```python
from build123d import *

# Parameters (mm, degrees)
F0_R     = 4.925
F0_W     = 15.85
F0_H     = 3
F0_H_2   = 14
F1_DEPTH = 3
F2_DEPTH = 60
F3_DEPTH = 10


with BuildPart() as f1:
    # F0 (on Top) → F1 (new body)
    with BuildSketch(Plane.XY):
        with BuildLine():
            Line((-7.925, 5.925), (-7.925, 0))
            ThreePointArc((-7.925, 0), (0, -7.925), (7.925, 0))
            Line((7.925, 0), (7.925, 5.925))
            Line((7.925, 5.925), (-7.925, 5.925))
        make_face()
        Circle(F0_R, mode=Mode.SUBTRACT)
        with Locations((0, 7.425)):
            Rectangle(F0_W, F0_H)
        with Locations((0, 15.925)):
            Rectangle(F0_W, F0_H_2)
        with Locations((0, 24.425)):
            Rectangle(F0_W, F0_H)
    extrude(amount=F1_DEPTH)

    # F0 (on Top) → F2 (join)
    with BuildSketch(Plane.XY):
        with Locations((0, 7.425)):
            Rectangle(F0_W, F0_H)
        with Locations((0, 24.425)):
            Rectangle(F0_W, F0_H)
    extrude(amount=F2_DEPTH)

    # F0 (on Top) → F3 (join)
    with BuildSketch(Plane.XY):
        with BuildLine():
            Line((-7.925, 5.925), (-7.925, 0))
            ThreePointArc((-7.925, 0), (0, -7.925), (7.925, 0))
            Line((7.925, 0), (7.925, 5.925))
            Line((7.925, 5.925), (-7.925, 5.925))
        make_face()
        Circle(F0_R, mode=Mode.SUBTRACT)
    extrude(amount=F3_DEPTH)


solid = f1.part
```
Geometry: final body of the model. Coordinates: model frame, mm. A direction names the side the tool comes from. Give positions to 0.01 mm unless a question says otherwise; leave off trailing zeros. Loops run counter-clockwise (first coordinate to the right, second up) from the corner with the lowest first, then second, coordinate; pieces in that order, holes last. Notation, with made-up numbers: (15, 39) - (20, 39) arc R33 ccw to (20, 72) - close; hole circle Ø11 at (56, 15.5). An arc over 180 degrees is marked (long way). Answer as CSV lines item,"result". Start each with the question number.
(1) Section query B-B (x = 0). Output: boundary loops of the cut face in (y, z) (3 decimals), and give its area (3 significant figures).
(2) Section query D-D (y = 2). Output: boundary loops of the cut face in (x, z) (3 decimals).
(3) Pin query (flat end, axial travel): P1, Ø6, axis at x = 5.5, y = 20, coming from the -Z side; P2, Ø3, axis at x = -4.5, y = 2.5, coming from the +Z side; P3, Ø4, axis at x = 4, z = 6, coming from the -Y side; P4, Ø5, axis at x = -3, z = 43, coming from the -Y side (3 decimals). Return the tip coordinate at first contact, or that it passes through.
(4) Ray query, line 1 along Y through (x, z) = (0, 3.5) (3 decimals); line 2 along Y through (x, z) = (6.25, 17) (3 decimals); line 3 along Y through (x, z) = (4, 8) (3 decimals). Return the intervals inside material, ascending. Write a range as [from, to].
(5) Section query A-A (z = 19.5). Output: boundary loops of the cut face in (x, y) (3 decimals), and give its area (3 significant figures).
(6) Section query C-C (z = 9). Output: boundary loops of the cut face in (x, y) (3 decimals), and give its area (3 significant figures).
(7) Mould query, pull axis Y, two halves, no side actions, for faces 1 (the face through (-7.925, 8, 25)), 2 (the face through (-0.174, -7.923, 4.93)), 3 (the face through (0, 22.925, 31)). Classes: +Y half, -Y half, draft (parallel to the pull), parting line (faces both ways), or undercut.
(8) Reachability of faces 4 (the face through (3.4, -4, 10)), 5 (the face through (0, 13, 0)), 6 (the face through (0, 16, 3)) from +Z, -Z, +X, -X, +Y, -Y: full face, straight path, thin tool, end or side. Return the list, or none.
Worked answers:
1,outline,"(-7.925, 0) - (-4.925, 0) - (-4.925, 10) - (-7.925, 10) - close; (4.925, 0) - (25.925, 0) - (25.925, 60) - (22.925, 60) - (22.925, 3) - (8.925, 3) - (8.925, 60) - (5.925, 60) - (5.925, 10) - (4.925, 10) - close"
1,area,"442 mm^2"
2,outline,"(-7.925, 0) - (-4.501, 0) - (-4.501, 10) - (-7.925, 10) - close; (4.501, 0) - (7.925, 0) - (7.925, 10) - (4.501, 10) - close"
3,P1,"stops at z = 0"
3,P2,"stops at z = 10"
3,P3,"stops at y = -7.67"
3,P4,"stops at y = 5.925"
4,line 1,"y = [-7.925, -4.925], [4.925, 8.925], [22.925, 25.925]"
4,line 2,"y = [5.925, 8.925], [22.925, 25.925]"
4,line 3,"y = [-6.841, -2.873], [2.873, 8.925], [22.925, 25.925]"
5,outline,"(-7.925, 5.925) - (7.925, 5.925) - (7.925, 8.925) - (-7.925, 8.925) - close; (-7.925, 22.925) - (7.925, 22.925) - (7.925, 25.925) - (-7.925, 25.925) - close"
5,area,"95.1 mm^2"
6,outline,"(-7.925, 0) arc R7.925 ccw to (7.925, 0) - (7.925, 8.925) - (-7.925, 8.925) - close; (-7.925, 22.925) - (7.925, 22.925) - (7.925, 25.925) - (-7.925, 25.925) - close; hole circle Ø9.85 at (0, 0)"
6,area,"211 mm^2"
7,face 1,"draft"
7,face 2,"-Y half"
7,face 3,"undercut"
8,face 4,"+Z, +X, -X, -Y"
8,face 5,"-Z, +X, -X, +Y, -Y"
8,face 6,"+Z, +X, -X"
